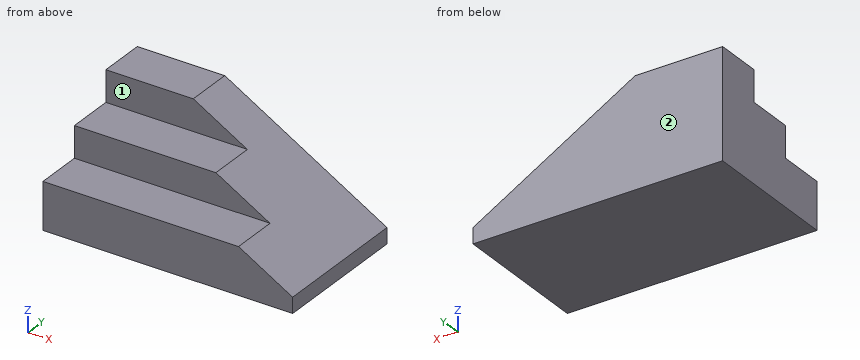
from build123d import *

# Parameters (mm, degrees)
F0_W     = 57.15
F0_H     = 6.35
F1_DEPTH = 101.6
F3_DEPTH = 57.15


with BuildPart() as f1:
    # F0 (on Right) → F1 (new body)
    with BuildSketch(Plane.YZ):
        Polygon((0, 6.35), (0, 44.45), (-19.05, 44.45), (-19.05, 31.75), (-38.1, 31.75), (-38.1, 19.05), (-57.15, 19.05), (-57.15, 6.35), align=None)
        with Locations((-28.575, 3.175)):
            Rectangle(F0_W, F0_H)
    extrude(amount=F1_DEPTH)

    # F2 (on Front) → F3 (cut)
    with BuildSketch(Plane.XZ):
        Polygon((101.6, 44.45), (35.56, 44.45), (101.6, 6.35), align=None)
    extrude(amount=F3_DEPTH, mode=Mode.SUBTRACT)


solid = f1.part
For this review, take the finished solid that the model builds, in its own axes (mm). Face numbers are marked on the shaded views. A direction names the side the tool comes from. Round coordinates to 2 decimals unless told otherwise and drop trailing zeros. Write each loop counter-clockwise with the first axis right and the second up, starting at its lowest first coordinate (ties: lowest second). Pieces come first, ordered by that corner, then holes. Notation, with made-up numbers: (61, -10) - (84, -10) arc R31 ccw to (84, 24) - close; hole circle Ø5 at (0.25, 54). An arc over 180 degrees is marked (long way). Write item = value, one per line. Start each with the question number.
1. For pin 1 Ø6 at (x, z) = (45, 21.5) entering from -Y; pin 2 Ø1.5 at (x, y) = (69, -40) entering from +Z; pin 3 Ø5.5 at (x, y) = (22.5, -32) entering from +Z; pin 4 Ø10 at (x, z) = (28, 37.5) entering from -Y, all flat-tipped, find the tip position at first contact; note any pin that passes through.
2. For the marked faces 1 and 2, list the 3-axis set-ups (+Z, -Z, +X, -X, +Y, -Y) from which the entire face can be reached by the end or side of a thin tool; tool diameter is ignored.
3. Consider section C-C on z = 9.5. State the section outline as (x, y) points, plus the area to 3 significant figures.
4. Consider section A-A on y = -33. State the section outline as (x, z) points.
5. Consider section D-D on x = 66.5. State the section outline as (y, z) points, plus the area to 3 significant figures.
6. Wall thickness on L1, parallel to Y at x = 46.5, z = 20; L2, parallel to Z at x = 15, y = -24.5; L3, parallel to Y at x = 27.5, z = 33.5: over which ranges is each line inside the solid? List them lowest first.
7. Consider section B-B on x = 17.5. State the section outline as (y, z) points, plus the area to 3 significant figures.
Evaluation:
q1.pin_1 = -57.15
q1.pin_2 = 19.05
q1.pin_3 = 31.75
q1.pin_4 = -19.05
q2.face_1 = +Z, +X, -X, -Y
q2.face_2 = +Z, -Z, +X, -X, +Y
q3.outline = (0, -57.15) - (96.14, -57.15) - (96.14, 0) - (0, 0) - close
q3.area = 5,490 mm2
q4.outline = (0, 0) - (101.6, 0) - (101.6, 6.35) - (57.57, 31.75) - (0, 31.75) - close
q5.outline = (-57.15, 0) - (0, 0) - (0, 26.6) - (-38.1, 26.6) - (-38.1, 19.05) - (-57.15, 19.05) - close
q5.area = 1,380 mm2
q6.L1 = -38.1 to 0
q6.L2 = 0 to 31.75
q6.L3 = -19.05 to 0
q7.outline = (-57.15, 0) - (0, 0) - (0, 44.45) - (-19.05, 44.45) - (-19.05, 31.75) - (-38.1, 31.75) - (-38.1, 19.05) - (-57.15, 19.05) - close
q7.area = 1,810 mm2
